CAD build for the part. Positions are in the model's coordinates, mm. Give positions to 0.01 mm unless a question says otherwise; leave off trailing zeros. Write each loop counter-clockwise with the first axis right and the second up, starting at its lowest first coordinate (ties: lowest second). Pieces come first, ordered by that corner, then holes. Notation, with made-up numbers: (-12, 50.25) -> (2, 50.25) arc R28 cw to (2, 87.25) -> close; hole circle Ø11 at (46, -30.5). An arc over 180 degrees is marked (long way). Answer as a JSON object with one key per item and string values.
Autodesk Inventor part; units mm, degrees
ref_plane "YZ Plane" through (0, 0, 0) normal (1, 0, 0) x (0, 1, 0)
ref_plane "XZ Plane" through (0, 0, 0) normal (0, 1, 0) x (-1, 0, 0)
ref_plane "XY Plane" through (0, 0, 0) normal (0, 0, 1) x (1, 0, 0)
sketch "Sketch1" plane through (0, 0, 0) normal (0, 1, 0) x (-1, 0, 0)
  line L0 (0, 0) -> (5.031, 0)
  line L1 (5.031, 0) -> (5.031, -10)
  line L2 (5.031, -10) -> (0, -10)
  line L3 (0, -10) -> (0, 0)
  dimension "d0" = 10
extrude "Extrusion1" add sketch "Sketch1" along normal blind 5
sketch "Sketch2" plane through (0, 5, 0) normal (0, 1, 0) x (1, 0, 0)
  point P0 (0, 0)
sketch "Sketch3" plane through (0, 5, 0) normal (0, 1, 0) x (1, 0, 0)
  circle A0 centre (-2.8935, 6.2146) radius 1
  point P0 (0, 0)
  dimension "d14" = 2
extrude "Extrusion2" cut sketch "Sketch3" against normal blind 5
fillet "Fillet1" radius 0.8 1 edges at (0, 2.5, 0)
chamfer "Chamfer1" distance 2 angle 45 1 edges at (0, 2.5, -10)
sketch "Sketch4" plane through (0, 5, 0) normal (0, 1, 0) x (1, 0, 0)
  line L0 (-5.031, 0) -> (-0.8, 0) construction
  line L1 (-5.031, 0) -> (-5.031, 5.2141) construction
  line L2 (-5.031, 5.2141) -> (-0.484, 5.2141) construction
  line L3 (-0.484, 5.2141) -> (-0.484, 0) construction
  line L4 (-0.484, 0) -> (-3.3034, 3.9743) construction
  line L5 (-3.3034, 3.9743) -> (-0.484, 5.2141) construction
  line L6 (-5.031, 0) -> (-5.031, 3) construction
  line L7 (-5.031, 10) -> (-5.031, 0) construction
  line L8 (-5.031, 3) -> (-2.031, 3) construction
  circle A0 centre (-2.031, 3) radius 1 construction
  circle A1 centre (-2.031, 3) radius 1
  point P0 (0, 0)
  dimension "d9" = 3
  dimension "d10" = 3
  dimension "d11" = 90
  dimension "d12" = 2
  dimension "d13" = 2
properties part number "testpart"
1) Slice it at C-C (x = -2.2). List the corners of the cut face in (y, z), then the cut area to 3 significant figures.
Model answer:
{"outline": "(0, -10) -> (5, -10) -> (5, -6.94) -> (0, -6.94) -> close; (0, -5.49) -> (5, -5.49) -> (5, 0) -> (0, 0) -> close", "area": "42.8 mm2"}
2) Slice it at B-B (y = 1.25). List the corners of the cut face in (x, z).
Model answer:
{"outline": "(-5.03, -10) -> (-2, -10) -> (0, -8) -> (0, -0.8) arc R0.8 ccw to (-0.8, 0) -> (-5.03, 0) -> close; hole circle Ø2 at (-2.89, -6.21)"}
3) Wall check: probe 1 along X at (y, z) = (3.3, -6.5); probe 2 along Z at (x, y) = (-3, 3.3); probe 3 along Z at (x, y) = (-3.2, 2.5). Give the ranges that are in metal, low to high.
Model answer:
{"probe 1": "x = -5.03 to -3.85, -1.94 to 0", "probe 2": "z = -10 to -7.21, -5.22 to 0", "probe 3": "z = -10 to -7.17, -5.26 to 0"}
4) Mould opens along Z. For faces 1 (the flat face through (-3, 2, 0)), 2 (the cylindrical face through (-1.94, 2.54, -6.51)), 3 (the flat face through (-4, 2, -10)), 4 (the flat face through (-2, 0, -5)) say: released by +Z, released by -Z, zero draft, split by the parting line, or undercut.
Model answer:
{"face 1": "released by +Z", "face 2": "undercut", "face 3": "released by -Z", "face 4": "zero draft"}
5) Slice it at A-A (x = -2.9). List the corners of the cut face in (y, z).
Model answer:
{"outline": "(0, -10) -> (5, -10) -> (5, -7.21) -> (0, -7.21) -> close; (0, -5.21) -> (5, -5.21) -> (5, 0) -> (0, 0) -> close"}
6) Slice it at D-D (x = -1.15). List the corners of the cut face in (y, z), then the cut area to 4 significant figures.
Model answer:
{"outline": "(0, -9.15) -> (5, -9.15) -> (5, 0) -> (0, 0) -> close", "area": "45.75 mm2"}
